Here's the drawing with two shaded views (mm, measured from the low corner). I have some questions. Coordinates: 2 decimals unless noted, no trailing zeros. Write each loop counter-clockwise with the first axis right and the second up, starting at its lowest first coordinate (ties: lowest second). Pieces come first, ordered by that corner, then holes.
Item 1: Thinking about a two-plate mould opening in Z: for the marked faces 1, 2 and 3, which applies, +Z half, -Z half, draft (parallel to the pull), parting line (faces both ways), or undercut?
Item 2: If I drill on probe 1 along Z at (x, y) = (14, 11); probe 2 along Y at (x, z) = (5, 4) (1 decimal); probe 3 along X at (y, z) = (8, 3.25), over which ranges is the centre line in solid material (lowest first)?
Item 3: I want a section at D-D on x = 8.5. Please give me the cut outline in (y, z).
Item 4: For P1, Ø8, axis at x = 8, z = 13, coming from the -Y side; P2, Ø5, axis at x = 32, y = 11.5, coming from the +Z side; P3, Ø5, axis at y = 32.5, z = 6.5, coming from the +X side (1 decimal); P4, Ø3, axis at x = 23, y = 19.5, coming from the -Z side, each with a flat end and sliding along its axis, tell me the tip position at first contact or that it passes through.
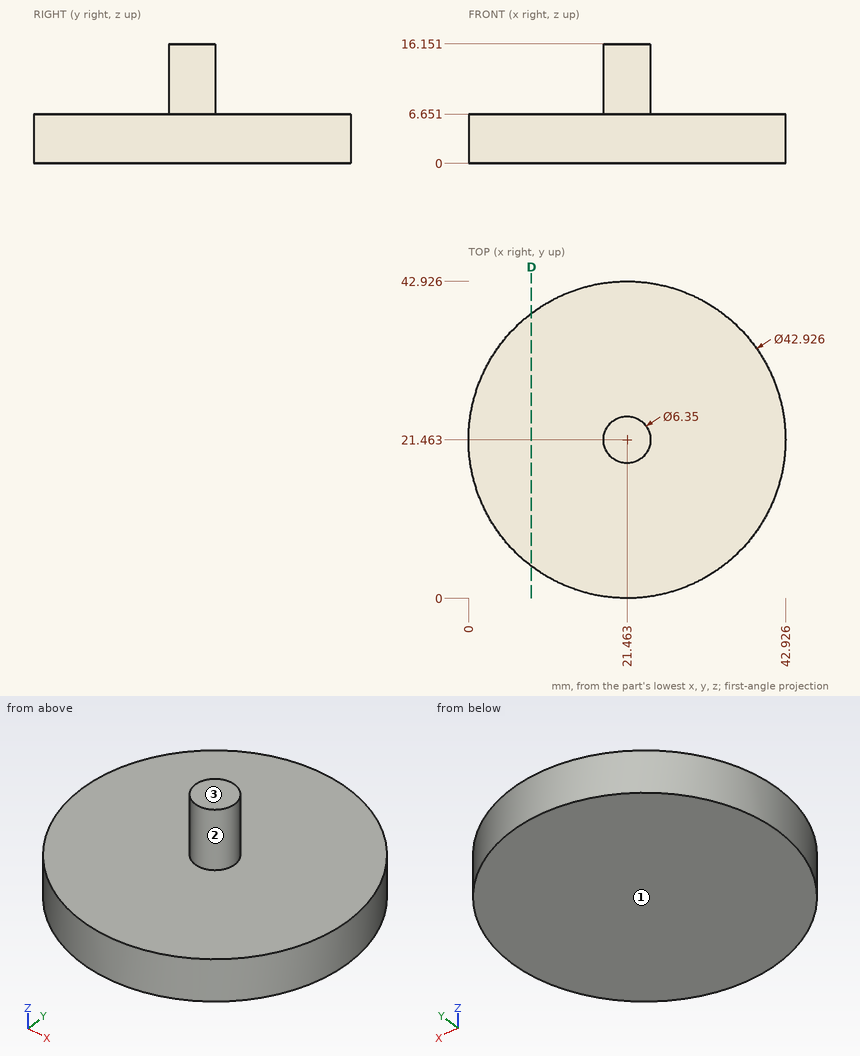
Response values:
1. face 1: -Z half
1. face 2: draft
1. face 3: +Z half
2. probe 1: z = 0 to 6.65
2. probe 2: y = 7.7 to 35.2
2. probe 3: x = 4.75 to 38.18
3. outline: (4.36, 0) - (38.57, 0) - (38.57, 6.65) - (4.36, 6.65) - close
4. P1: passes through
4. P2: stops at z = 6.65
4. P3: stops at x = 41.2
4. P4: stops at z = 0
